Autodesk Inventor part; units mm, degrees
ref_plane "Work Plane1" through (29, 0, 0) normal (0, -1, 0) x (1, 0, 0)
ref_plane "YZ Plane" through (0, 0, 0) normal (1, 0, 0) x (0, 1, 0)
ref_plane "XZ Plane" through (0, 0, 0) normal (0, 1, 0) x (-1, 0, 0)
sketch "Sketch1" plane through (0, 0, 0) normal (0, 0, 1) x (1, 0, 0)
  line L0 (-0.0667, 0) -> (20, 0)
  line L1 (20, 0) -> (20, 2)
  line L2 (20, 2) -> (2.1, 2)
  line L3 (2.1, 2) -> (1.6705, 2)
  line L4 (1.6705, 2) -> (0, 2)
  line L5 (0, 2) -> (0, 3.8)
  line L6 (0, 3.8) -> (-2.2, 3.8)
  line L7 (-2.2, 3.8) -> (-2.2, 1.4434)
  line L8 (-2.2, 1.4434) -> (-0.9, 1.4434)
  line L9 (-0.9, 1.4434) -> (-0.0667, 0)
  line L10 (-6.64, 0) -> (24.44, 0)
  line L11 (0, -0.76) -> (0, 4.56)
  line L12 (2.1, 2) -> (0, 2) construction
  dimension "d1" = 17.9
  dimension "d2" = 0.4295
  dimension "d3" = 2.2
  dimension "d4" = 1.3
  dimension "d5" = 60
  dimension "d6" = 4
  dimension "d7" = 4
  dimension "d8" = 2.8868
  dimension "d9" = 7.6
  dimension "d26" = 20
revolve "Body" add sketch "Sketch1" angle 360 about axis through (-0.0667, 0, 0) along (1, 0, 0)
sketch "Sketch2" plane through (-2.2, 0, 0) normal (-1, 0, 0) x (0, 0, 1)
  circle A0 centre (0, 0) radius 1.4434
  line L0 (0, -5.32) -> (0, 5.32)
  line L1 (-5.32, 0) -> (5.32, 0)
  line L2 (1.4434, 0) -> (0.7217, -1.25)
  line L3 (0.7217, -1.25) -> (-0.7217, -1.25)
  line L4 (-0.7217, -1.25) -> (-1.4434, 0)
  line L5 (-1.4434, 0) -> (-0.7217, 1.25)
  line L6 (-0.7217, 1.25) -> (0.7217, 1.25)
  line L7 (0.7217, 1.25) -> (1.4434, 0)
  point P0 (0, 0)
extrude "Slot" add sketch "Sketch2" against normal up to next contours L7 A0 | A0 L2 | L6 L0 A0 | A0 L0 L3 | L0 L6 A0 | A0 L3 L0 | L4 A0 | A0 L5
fillet "Fillet1" radius 1.9 1 edges at (-2.2, -3.8, 0)
thread "Thread"
chamfer "Chamfer1" distance 0.4294 distance2 0.4294 1 edges at (20, -2, 0) measured on face at (20, 0.527, -0.2661)
ref_plane "Work Plane1" through (29, 0, 0) normal (0, -1, 0) x (1, 0, 0)
fillet "Fillet2" radius 0.4 1 edges at (0, -2, 0)
equation "\"d1\" = GEL"
equation "\"d3\" = KOH"
equation "\"d4\" = INTI"
equation "\"d6\" = GD"
equation "\"d7\" = BDM"
equation "\"d8\" = 1.1547 * SW"
equation "\"d9\" = KOD"
equation "\"d26\" = NLG"
equation "\"d30\" = R"
equation "\"d17\" = RR"
equation "\"d13\" = GEL"
equation "\"d15\" = -0.5 * SPD + 0.5 * GD"
equation "\"d16\" = GUL"
equation "\"GD\" = NND"
equation "\"NLG\" = 20"
equation "\"GEL\" = 17.9"
equation "\"KOD\" = 7.6"
equation "\"KOH\" = 2.2"
equation "\"INTI\" = 1.3"
equation "\"GAL\" = 0.61345 * PTC"
equation "\"GUL\" = 0.61345 * PTC"
equation "\"BDM\" = NND"
equation "\"SW\" = 2.5"
equation "\"RR\" = 1.9"
equation "\"SPD\" = NND - 1.2269 * PTC"
equation "\"R\" = 0.4"
equation "\"TOA\" = 30deg"
equation "\"GD1\" = THREADDIA - 1.2269 * PTC"
equation "\"THREADDIA\" = 4"
equation "\"PTC\" = 0.7"
equation "\"NND\" = 4"
equation "\"KOH1\" = 0.3"
equation "\"E0\" = 2.873"
properties part number "ISO 7380-1 - M4 x 20" material "Steel"
Model file for the job. Use its own axes, mm. A direction names the side the tool comes from. Give positions to 0.01 mm unless a question says otherwise; leave off trailing zeros. Order: outer loops, then holes, each group sorted by start corner. A loop starts at its lowest first (then second) coordinate and runs counter-clockwise, first axis right, second up. Notation, with made-up numbers: M 46.25,60.5 L 85.25,60.5 A19 cw 85.25,67.5 Z; hole C -21,63.25 d4. An arc over 180 degrees is marked long. Write item = value, one per line.
Q1. Drill centre lines: line 1 (Y direction, x = 11.5, z = 1.75); line 2 (Z direction, x = 9.25, y = 0.5); line 3 (X direction, y = 3.25, z = 0.25). Where is each one in solid material? Low to high. Write a range as [from, to].
Derived:
line_1 = [-0.97, 0.97]
line_2 = [-1.94, 1.94]
line_3 = [-1.63, 0]
Q2. Two-plate mould, pull along Z, no slides. Class faces 1 (the cylindrical face through (-0.15, -2.8, -2.57)), 2 (the flat face through (0, 2.5, -0.8)), 3 (the flat face through (-1.504, 0.616, -1.088)): pulls with the +Z half, pulls with the -Z half, needs draft (parallel to the pull), parting line crosses it, or undercut.
Derived:
face_1 = parting line crosses it
face_2 = needs draft
face_3 = undercut
Q3. Cut at A-A, the plane x = 4.25. List the corners of the cut face in (y, z), then the cut area to 3 significant figures.
Derived:
outline = C 0,0 d4
area = 12.6 mm2
Q4. Tool access for faces 4 (the flat face through (-1.504, -0.616, 1.088)), 5 (the cylindrical face through (10, 0, 2)), 6 (the flat face through (20, 0, 0)): list every direction of +Z, -Z, +X, -X, +Y, -Y with a clear straight run to the whole face (end or side of a thin tool).
Derived:
face_4 = -X
face_5 = +X
face_6 = +Z, -Z, +X, +Y, -Y
Q5. Flat gauge pins, fed straight in: pin 1 (3 mm diameter, centred on y = 1.5, z = -1.5, fed in from -X); pin 2 (2 mm diameter, centred on x = 9.5, z = 2, fed in from -Y); pin 3 (3 mm diameter, centred on x = 10, z = 0, fed in from +Y); pin 4 (3 mm diameter, centred on x = 12.5, y = 2, fed in from -Z). Where does each tip first touch, or does it go through?
Derived:
pin_1 = -2.2
pin_2 = -1.73
pin_3 = 2
pin_4 = -1.94
